Geometry check sheet. Reference: the model listing, model coordinates, mm. Give positions to 0.01 mm unless a question says otherwise; leave off trailing zeros. Order: outer loops, then holes, each group sorted by start corner. A loop starts at its lowest first (then second) coordinate and runs counter-clockwise, first axis right, second up.
from build123d import *

# Parameters (mm, degrees)
EXTRUDE1_DEPTH            = 3.2
SKETCH5_R                 = 6.5
CHASSIS_MOUNT_HOLES_DEPTH = 244.405812041
SKETCH6_R                 = 4.5
ENGINE_MOUNT_HOLES_DEPTH  = 244.405812041


with BuildPart() as part:
    # Sketch4 → Extrude1 (new body)
    with BuildSketch(Plane(origin=(0, 0, 0), x_dir=(0, 0, -1), z_dir=(1, 0, 0))):
        with BuildLine():
            Line((62.532051611, 158.051475499), (157.209419868, 171.960961445))
            ThreePointArc((157.209419868, 171.960961445), (171.960961445, 160.988631666), (160.988631666, 146.237090089))
            Line((160.988631666, 146.237090089), (83.804641545, 134.897636473))
            ThreePointArc((83.804641545, 134.897636473), (81.285036333, 134.84841996), (78.833134949, 135.430667579))
            ThreePointArc((78.833134949, 135.430667579), (57.476451891, 135.335862335), (41.594586736, 121.057092835))
            ThreePointArc((41.594586736, 121.057092835), (40.693699631, 119.560345202), (39.600266647, 118.197900576))
            ThreePointArc((39.600266647, 118.197900576), (21.5857968, 86.934366989), (18.660417288, 50.97088814))
            Line((18.660417288, 50.97088814), (22.745312053, 21.905351613))
            ThreePointArc((22.745312053, 21.905351613), (22.700845783, 17.796400072), (21.440584589, 13.88523634))
            Line((21.440584589, 13.88523634), (11.636162946, -5.796526027))
            ThreePointArc((11.636162946, -5.796526027), (-3.307639706, -12.572172512), (-12.982184032, 0.680367435))
            Line((-12.982184032, 0.680367435), (-11.728287792, 24.606132992))
            ThreePointArc((-11.728287792, 24.606132992), (-11.013879957, 26.397161442), (-9.356926136, 27.383399496))
            ThreePointArc((-9.356926136, 27.383399496), (4.476016858, 43.584120766), (-7.587711328, 61.142029063))
            ThreePointArc((-7.587711328, 61.142029063), (-9.132498235, 62.296063238), (-9.655779017, 64.1519562))
            ThreePointArc((-9.655779017, 64.1519562), (-0.849075896, 102.602883239), (20.462203873, 135.797177398))
            ThreePointArc((20.462203873, 135.797177398), (39.583099322, 150.54263352), (62.532051611, 158.051475499))
        make_face()
    extrude(amount=EXTRUDE1_DEPTH)

    # Sketch5 → chassis mount holes (cut, through all)
    with BuildSketch(Plane(origin=(0, 0, 0), x_dir=(0, 0, -1), z_dir=(1, 0, 0))):
        Circle(SKETCH5_R)
        with Locations((159.099025767, 159.099025767)):
            Circle(SKETCH5_R)
        with Locations((30.03123526, 126.997538987)):
            Circle(SKETCH5_R)
    extrude(amount=CHASSIS_MOUNT_HOLES_DEPTH, mode=Mode.SUBTRACT)

    # Sketch6 → engine mount holes (cut, through all)
    with BuildSketch(Plane(origin=(0, 0, 0), x_dir=(0, 0, -1), z_dir=(1, 0, 0))):
        with Locations((9.170519858, 19.997538987)):
            Circle(SKETCH6_R)
        with Locations((92.049906905, 148.605498316)):
            Circle(SKETCH6_R)
    extrude(amount=ENGINE_MOUNT_HOLES_DEPTH, mode=Mode.SUBTRACT)


solid = part.part
Item 1: Sectioned sample at B-B (z = 0). Enter the section's corners in (x, y), and give its area (3 significant figures).
Reported:
outline: (0, -13) - (3.2, -13) - (3.2, -6.5) - (0, -6.5) - close; (0, 6.5) - (3.2, 6.5) - (3.2, 32.78) - (0, 32.78) - close; (0, 56.22) - (3.2, 56.22) - (3.2, 104.57) - (0, 104.57) - close
area: 260 mm2
Item 2: Draft check along Y on faces 1 (the flat face through (1.578, 36.642, -20.674)), 2 (the flat face through (1.58, 164.91, -109.21)), 3 (the flat face through (1.578, 4.182, -16.607)). Enter one of: released by +Y, released by -Y, zero draft, split by the parting line, or undercut.
Reported:
face 1: undercut
face 2: released by +Y
face 3: released by -Y
Item 3: Sectioned sample at C-C (y = 67). Enter the section's corners in (x, z), and give its area (3 significant figures).
Reported:
outline: (0, -17.99) - (3.2, -17.99) - (3.2, 9.47) - (0, 9.47) - close
area: 87.9 mm2
Item 4: Sectioned sample at D-D (z = -143.5). Enter the section's corners in (x, y).
Reported:
outline: (0, 143.67) - (3.2, 143.67) - (3.2, 169.95) - (0, 169.95) - close
Item 5: Scan lines: L1, parallel to Y at x = 2.35, z = 0; L2, parallel to Z at x = 0.55, y = 64; L3, parallel to Z at x = 2.95, y = 5. Record each from-to range of solid material in increasing order.
Reported:
L1: y = -13 to -6.5, 6.5 to 32.78, 56.22 to 104.57
L2: z = -17.87 to 9.66
L3: z = -17.01 to -4.15, 4.15 to 12.76
Item 6: Sectioned sample at A-A (x = 0.55). Enter the section's corners in (y, z), and give its area (3 significant figures).
Reported:
outline: (-5.8, -11.64) - (13.89, -21.44) arc R13.71 ccw to (21.91, -22.75) - (50.97, -18.66) arc R82.38 cw to (118.2, -39.6) arc R13 ccw to (121.06, -41.59) arc R30 cw to (135.43, -78.83) arc R10 ccw to (134.9, -83.8) - (146.24, -160.99) arc R13 ccw to (171.96, -157.21) - (158.05, -62.53) arc R71.22 ccw to (135.8, -20.46) arc R114.71 ccw to (64.15, 9.66) arc R3 ccw to (61.14, 7.59) arc R17.5 cw to (27.38, 9.36) arc R3 ccw to (24.61, 11.73) - (0.68, 12.98) arc R13 ccw to start; hole circle Ø13 at (0, 0); hole circle Ø9 at (20, -9.17); hole circle Ø13 at (127, -30.03); hole circle Ø9 at (148.61, -92.05); hole circle Ø13 at (159.1, -159.1)
area: 6,810 mm2
